Can you work these out from the drawing? Everything is in mm from the part's minimum corner. A direction names the side the tool comes from. Give positions to 0.01 mm unless a question says otherwise; leave off trailing zeros. Order: outer loops, then holes, each group sorted by start corner. A loop starts at its lowest first (then second) coordinate and runs counter-clockwise, first axis right, second up. Notation, with made-up numbers: M 7.5,-12.75 L 28.5,-12.75 A21 ccw 28.5,11.25 Z; hole C -7.5,-36.75 d8. An arc over 180 degrees is marked long. Answer in a Markdown table with one row per item. Add a question column.
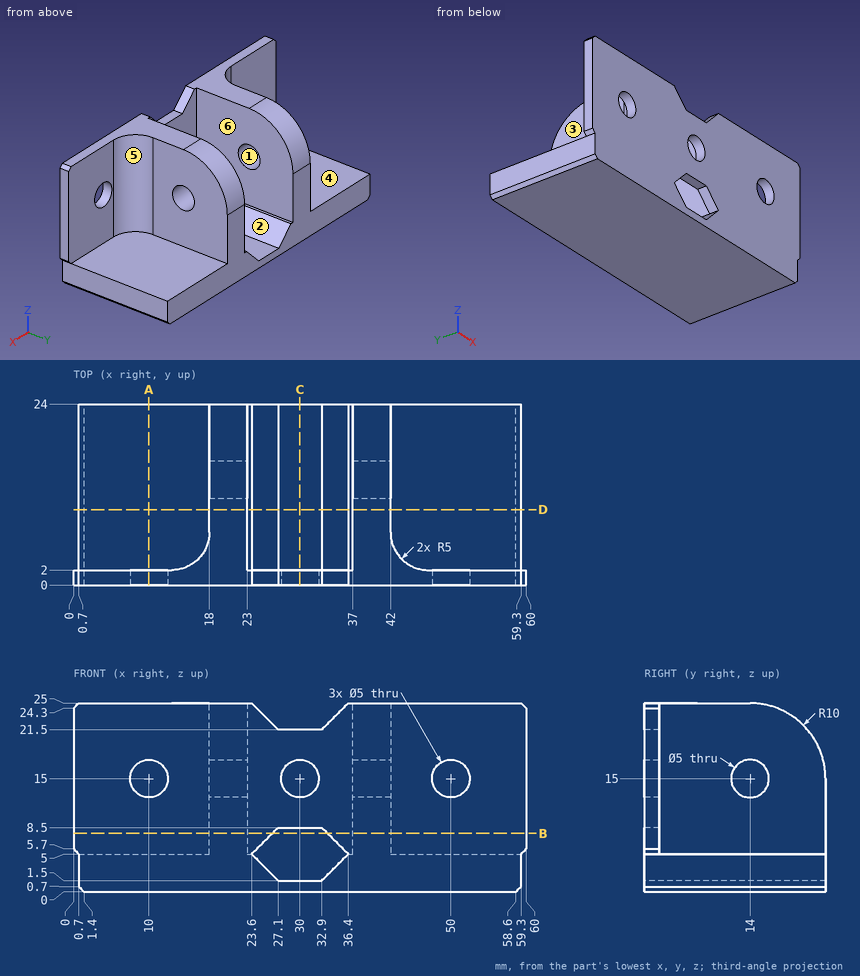
1. Thinking about a two-plate mould opening in X: for the marked faces 1, 2 and 3, which applies, pulls with the +X half, pulls with the -X half, needs draft (parallel to the pull), parting line crosses it, or undercut?
2. For the marked faces 4, 5 and 6, which set-ups out of +Z, -Z, +X, -X, +Y, -Y let a thin tool reach every point of the face, with its end or its side?
3. Suppose I cut it at B-B on z = 7.75. List the corners of the cut face in (x, y) for me.
4. Suppose I cut it at C-C on x = 30. List the corners of the cut face in (y, z) for me, plus the area to 3 significant figures.
5. Will these pins go through, and if not, where does the flat tip stop? P1, Ø1, axis at y = 6, z = 8, coming from the +X side; P2, Ø2, axis at y = 11, z = 18, coming from the -X side; P3, Ø4, axis at x = 27, z = 19, coming from the +Y side.
6. If I drill on line 1 along X through (y, z) = (1.2, 15); line 2 along X through (y, z) = (10.5, 15); line 3 along Y through (x, z) = (9, 19.75), over which ranges is the centre line in solid material (lowest first)? Write a range as [from, to].
7. Suppose I cut it at A-A on x = 10. List the corners of the cut face in (y, z) for me, plus the area to 3 significant figures.
8. Suppose I cut it at D-D on y = 10. List the corners of the cut face in (x, z) for me, plus the area to 3 significant figures.
Findings below:
| question | item | result |
|---|---|---|
| 1 | face 1 | needs draft |
| 1 | face 2 | undercut |
| 1 | face 3 | pulls with the -X half |
| 2 | face 4 | +Z, -X, +Y |
| 2 | face 5 | +Z, +X, +Y |
| 2 | face 6 | +Z, +Y |
| 3 | outline | M 0,0 L 26.35,0 L 26.35,2 L 23,2 L 23,24 L 18,24 L 18,7 A5 cw 13,2 L 0,2 Z; M 33.65,0 L 60,0 L 60,2 L 47,2 A5 cw 42,7 L 42,24 L 37,24 L 37,2 L 33.65,2 Z |
| 4 | outline | M 0,0 L 24,0 L 24,1.5 L 0,1.5 Z; M 0,8.5 L 2,8.5 L 2,12.5 L 0,12.5 Z; M 0,17.5 L 2,17.5 L 2,21.5 L 0,21.5 Z |
| 4 | area | 52.0 mm2 |
| 5 | P1 | x = 42.23 |
| 5 | P2 | x = 18 |
| 5 | P3 | y = 2 |
| 6 | line 1 | [0, 7.5], [12.5, 27.5], [32.5, 47.5], [52.5, 60] |
| 6 | line 2 | [18, 23], [37, 42] |
| 6 | line 3 | [0, 2] |
| 7 | outline | M 0,0 L 24,0 L 24,5 L 2,5 L 2,12.5 L 0,12.5 Z; M 0,17.5 L 2,17.5 L 2,25 L 0,25 Z |
| 7 | area | 150 mm2 |
| 8 | outline | M 0.7,0.7 L 1.4,0 L 58.6,0 L 59.3,0.7 L 59.3,5 L 42,5 L 42,25 L 37,25 L 37,5 L 36.4,5 L 32.9,1.5 L 27.1,1.5 L 23.6,5 L 23,5 L 23,25 L 18,25 L 18,5 L 0.7,5 Z |
| 8 | area | 460 mm2 |
